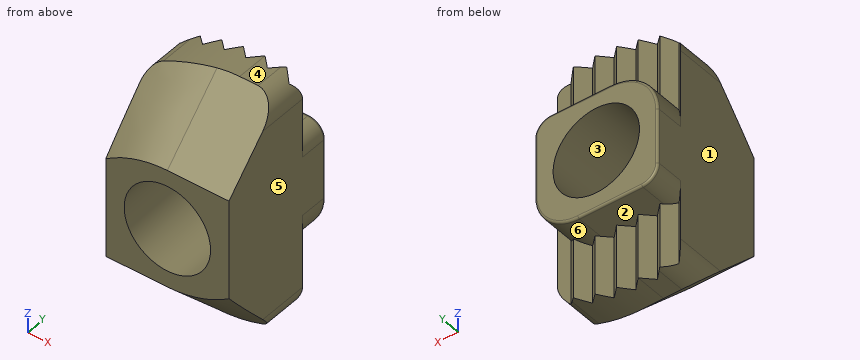
```python
from build123d import *

# Parameters (mm, degrees)
EXTRUDE1_DEPTH          = 4.5
CUT_EXTRUDE1_DEPTH      = 8
CUT_EXTRUDE1_DEPTH_BACK = 8
CUT_EXTRUDE2_DEPTH      = 4
CUT_EXTRUDE2_DEPTH_BACK = 4
CUT_REVOLVE1_ANGLE      = 60
CUT_REVOLVE2_ANGLE      = 60
EXTRUDE2_START          = -0.2
SKETCH7_R               = 2
EXTRUDE2_DEPTH          = 5.5
SKETCH10_R              = 2
CUT_EXTRUDE4_DEPTH      = 6.7000001
FILLET1_R               = 0.1


with BuildPart() as part:
    # Sketch1 → Extrude1 (new body)
    with BuildSketch(Plane(origin=(0, 0, 0), x_dir=(1, 0, 0), z_dir=(0, 1, 0))):
        with BuildLine():
            Line((-1.85, 3.5), (-1, 3.5))
            ThreePointArc((-1, 3.5), (0.66503344, 3.324810774), (2.2571429, 2.806915911))
            ThreePointArc((2.2571429, 2.806915911), (2.688791661, 2.438003962), (2.85, 1.893551439))
            Line((2.85, 1.893551439), (2.85, -1.946775719))
            Line((2.85, -1.946775719), (2.85, -7))
            ThreePointArc((2.85, -7), (2.557106781, -7.707106781), (1.85, -8))
            Line((1.85, -8), (1, -8))
            ThreePointArc((1, -8), (-0.66503344, -7.824810774), (-2.2571429, -7.306915911))
            ThreePointArc((-2.2571429, -7.306915911), (-2.688791661, -6.938003962), (-2.85, -6.393551439))
            Line((-2.85, -6.393551439), (-2.85, -1.946775719))
            Line((-2.85, -1.946775719), (-2.85, 2.5))
            ThreePointArc((-2.85, 2.5), (-2.557106781, 3.207106781), (-1.85, 3.5))
        make_face()
    extrude(amount=EXTRUDE1_DEPTH)

    # Sketch2 → Cut-Extrude1 (cut, two sides)
    with BuildSketch(Plane.XY) as cut_extrude1_sk:
        Polygon((-4, 4.5), (-3.5, 4), (-3, 4.5), (-2.5, 4), (-2, 4.5), (-1.5, 4), (-1, 4.5), (-0.5, 4), (0, 4.5), (0.5, 4), (1, 4.5), (1.5, 4), (2, 4.5), (2.5, 4), (3, 4.5), (3.5, 4), (4, 4.5), (4, 5.5), (-4, 5.5), align=None)
    extrude(amount=CUT_EXTRUDE1_DEPTH, mode=Mode.SUBTRACT)
    extrude(cut_extrude1_sk.sketch, amount=-CUT_EXTRUDE1_DEPTH_BACK, mode=Mode.SUBTRACT)

    # Sketch4 → Cut-Extrude2 (cut, two sides)
    with BuildSketch(Plane(origin=(0, 0, 0), x_dir=(0, 0, -1), z_dir=(1, 0, 0))) as cut_extrude2_sk:
        Polygon((4.5, -1), (4.5, 4), (0.5, 0), (-5, 0), (-9, 4), (-9, -1), align=None)
    extrude(amount=CUT_EXTRUDE2_DEPTH, mode=Mode.SUBTRACT)
    extrude(cut_extrude2_sk.sketch, amount=-CUT_EXTRUDE2_DEPTH_BACK, mode=Mode.SUBTRACT)

    # Sketch5 → Cut-Revolve1 (revolve, cut)
    with BuildSketch(Plane(origin=(0, 0, 0), x_dir=(0, 0, -1), z_dir=(1, 0, 0))):
        Polygon((0, -1), (-9, -1), (-9, 3), (-8, 3), (-5, 0), (0, 0), align=None)
    revolve(axis=Axis((0, 3, 0), (0, -1, 0)), revolution_arc=CUT_REVOLVE1_ANGLE, mode=Mode.SUBTRACT)

    # Sketch6 → Cut-Revolve2 (revolve, cut)
    with BuildSketch(Plane(origin=(0, 0, 0), x_dir=(0, 0, -1), z_dir=(1, 0, 0))):
        Polygon((4.5, -1), (4.5, 3), (3.5, 3), (0.5, 0), (-4.5, 0), (-4.5, -1), align=None)
    revolve(axis=Axis((0, 3, 4.5), (0, -1, 0)), revolution_arc=CUT_REVOLVE2_ANGLE, mode=Mode.SUBTRACT)

    # Sketch7 → Extrude2 (add)
    with BuildSketch(Plane.XZ.offset(EXTRUDE2_START)):
        with BuildLine():
            Line((2.1, 5), (-0.65, 5))
            ThreePointArc((-0.65, 5), (-2.205634919, 4.355634919), (-2.85, 2.8))
            Line((-2.85, 2.8), (-2.85, 0.25))
            ThreePointArc((-2.85, 0.25), (-2.630330086, -0.280330086), (-2.1, -0.5))
            Line((-2.1, -0.5), (0.85, -0.5))
            ThreePointArc((0.85, -0.5), (2.264213562, 0.085786438), (2.85, 1.5))
            Line((2.85, 1.5), (2.85, 4.25))
            ThreePointArc((2.85, 4.25), (2.630330086, 4.780330086), (2.1, 5))
        make_face()
        with Locations((0, 2.25)):
            Circle(SKETCH7_R, mode=Mode.SUBTRACT)
    extrude(amount=-EXTRUDE2_DEPTH)

    # Sketch10 → Cut-Extrude4 (cut, through all)
    with BuildSketch(Plane(origin=(0, 5.7, 0), x_dir=(1, 0, 0), z_dir=(0, 1, 0))):
        with Locations((0, -2.25)):
            Circle(SKETCH10_R)
    extrude(amount=-CUT_EXTRUDE4_DEPTH, mode=Mode.SUBTRACT)

    # Fillet1
    fillet1_edges = [part.edges().sort_by_distance(p)[0] for p in [
        (-2.205634919, 5.7, 4.355634919),
        (0.725, 5.7, 5),
        (2.630330086, 5.7, 4.780330086),
        (2.85, 5.7, 2.875),
        (2.264213562, 5.7, 0.085786438),
        (-0.625, 5.7, -0.5),
        (-2.630330086, 5.7, -0.280330086),
        (-2.85, 5.7, 1.525),
    ]]
    fillet(fillet1_edges, radius=FILLET1_R)


solid = part.part
```
The listing builds one solid part. Answer for the finished solid, in the listing's coordinates (mm). Face numbers are marked on the shaded views. A direction names the side the tool comes from. Give positions to 0.01 mm unless a question says otherwise; leave off trailing zeros. Write each loop counter-clockwise with the first axis right and the second up, starting at its lowest first coordinate (ties: lowest second). Pieces come first, ordered by that corner, then holes. Notation, with made-up numbers: (-4.5, -11.75) - (41.5, -11.75) arc R34 ccw to (41.5, 26.25) - close; hole circle Ø5 at (-16, -31.5). An arc over 180 degrees is marked (long way). Use one line per item in the form item = value. Start each with the question number.
1) Find section C-C on y = 0.8. Determine the outline of the cut face in (x, z).
2) Find section B-B on y = 3.6. Determine the outline of the cut face in (x, z).
3) Flat-ended cylindrical pins translate along their axes: pin 1 Ø3 at (x, z) = (0, 2.25) entering from -Y; pin 2 Ø3 at (x, y) = (-2, 3) entering from +Z. Find the tip coordinate at first contact, or state that the pin passes through.
4) A tool of negligible diameter and unlimited length cuts with its end or side. For the marked faces 1 and 2, from which of +Z, -Z, +X, -X, +Y, -Y can it reach the whole face along a straight path? Write none if from no direction.
5) Find section A-A on z = 2.25. Determine the outline of the cut face in (x, y), plus the area to 3 significant figures.
6) Find section D-D on y = 2.3. Determine the outline of the cut face in (x, z), plus the area to 3 significant figures.
7) Consider line 1 along X through (y, z) = (3.65, 2.25); line 2 along Z through (x, y) = (0, 4.1); line 3 along Z through (x, y) = (0, 2.75). Determine where each line is inside the solid, lowest interval first. Write a range as from..to.
8) The mould has two halves that part along Z. Classify the marked faces 3, 4, 5 and 6: pulls with the +Z half, pulls with the -Z half, needs draft (parallel to the pull), parting line crosses it, or undercut.
Geometry results:
q1.outline = (-2.85, -1.3) - (0, -1.3) arc R5.8 ccw to (2.85, -0.55) - (2.85, 5.8) - (0, 5.8) arc R5.8 ccw to (-2.85, 5.05) - close; hole circle Ø4 at (0, 2.25)
q2.outline = (-2.85, -2.5) arc R1 ccw to (-1.85, -3.5) - (-1, -3.5) arc R8 ccw to (2.26, -2.81) arc R1 ccw to (2.85, -1.89) - (2.85, 7) arc R1 ccw to (1.85, 8) - (1, 8) arc R8 ccw to (-2.26, 7.31) arc R1 ccw to (-2.85, 6.39) - close; hole circle Ø4 at (0, 2.25)
q3.pin_1 = through
q3.pin_2 = 7.86
q4.face_1 = +Z, -Z, -X, +Y, -Y
q4.face_2 = -Z, +Y
q5.outline = (-2.85, 0) - (-2, 0) - (-2, 5.7) - (-2.75, 5.7) arc R0.1 ccw to (-2.85, 5.6) - close; (2, 0) - (2.85, 0) - (2.85, 5.6) arc R0.1 ccw to (2.75, 5.7) - (2, 5.7) - close
q5.area = 9.69 mm2
q6.outline = (-2.85, -2.5) arc R1 ccw to (-2.8, -2.8) - (0, -2.8) arc R7.3 ccw to (2.79, -2.25) arc R1 ccw to (2.85, -1.89) - (2.85, 7) arc R1 ccw to (2.8, 7.3) - (0, 7.3) arc R7.3 ccw to (-2.79, 6.75) arc R1 ccw to (-2.85, 6.39) - close; hole circle Ø4 at (0, 2.25)
q6.area = 43.9 mm2
q7.line_1 = -2.85..-2, 2..2.85
q7.line_2 = -3.44..0.25, 4.25..7.94
q7.line_3 = -3.25..0.25, 4.25..7.75
q8.face_3 = undercut
q8.face_4 = pulls with the +Z half
q8.face_5 = needs draft
q8.face_6 = pulls with the -Z half
